The model under review builds one solid part; all positions refer to its coordinate system, in mm. A direction names the side the tool comes from. Coordinates: 2 decimals unless noted, no trailing zeros. Order: outer loops, then holes, each group sorted by start corner. A loop starts at its lowest first (then second) coordinate and runs counter-clockwise, first axis right, second up. Notation, with made-up numbers: (75.5, 33.5) -> (89.5, 33.5) arc R26 cw to (89.5, 59.5) -> close; hole circle Ø4 at (10.5, 60.25). An arc over 180 degrees is marked (long way). Use one line per item in the form item = value. Start each with the question number.
(1) Mouldability with a two-part tool opening along X and no side actions: class faces 1 (the flat face through (-8.72, -8.47, -1.57)), 2 (the flat face through (8.47, -8.72, -1.57)), 3 (the flat face through (-6.26, -1.95, -1.57)) as +X half, -X half, draft (parallel to the pull), parting line (faces both ways), or undercut.
(2) Insertion check: pin 1 Ø5 at (x, y) = (5, -14.5) entering from +Z; pin 2 Ø1.5 at (y, z) = (1.5, 22.5) entering from +X; pin 3 Ø4 at (y, z) = (-1, 6.5) entering from +X. Each pin has a flat end and moves straight along its axis. Give the tip position at first contact, or say it passes through.
(3) Take a section at A-A (y = -3). State the section outline as (x, z) points (3 decimals).
(4) Wall thickness on line 1 along Z through (x, y) = (-13, 2.5) (3 decimals); line 2 along X through (y, z) = (-0.5, 25.5); line 3 along Y through (x, z) = (9.5, 35): over which ranges is each line inside the solid? List them lowest first.
(5) Take a section at B-B (y = 2.5). State the section outline as (x, z) points (3 decimals), then the cut area to 3 significant figures.
(6) For faces 4 (the flat face through (6.44, -1.77, -1.57)), 5 (the flat face through (-14.91, 2.28, -1.57)), list the 3-axis set-ups (+Z, -Z, +X, -X, +Y, -Y) from which the entire face can be reached by the end or side of a thin tool; tool diameter is ignored.
(7) Take a section at C-C (x = 15). State the section outline as (y, z) points (3 decimals).
(8) Take a section at D-D (y = -15.25). State the section outline as (x, z) points (3 decimals).
```python
from build123d import *

# Parameters (mm, degrees)
F1_R     = 1.651
F4_DEPTH = 3.175


with BuildPart() as f2:
    # F2: sweep along a path in F0
    with BuildLine(Plane.XZ) as f2_path:
        Line((-12.7, 0), (-7.687481, 40.823691))
        ThreePointArc((-7.687481, 40.823691), (0, 47.625), (7.687481, 40.823691))
        Line((7.687481, 40.823691), (12.7, 0))
    # F1 (on Top) → F2 (sweep)
    with BuildSketch(Plane.XY):
        with Locations((-12.7, 0)):
            Circle(F1_R)
    sweep(path=f2_path.line)

    # F3 (on Top) → F4 (join)
    with BuildSketch(Plane.XY):
        Polygon((-17.190128, 0), (0, -17.190128), (0, -8.209872), (-12.7, 4.490128), align=None)
        Polygon((0, -8.209872), (0, -17.190128), (17.190128, 0), (12.7, 4.490128), align=None)
    extrude(amount=-F4_DEPTH)


solid = f2.part
```
Findings:
q1.face_1 = -X half
q1.face_2 = +X half
q1.face_3 = undercut
q2.pin_1 = 0
q2.pin_2 = 11.42
q2.pin_3 = 13.77
q3.outline = (-14.19, -3.175) -> (-5.21, -3.175) -> (-5.21, 0) -> (-14.19, 0) -> close; (5.21, -3.175) -> (14.19, -3.175) -> (14.19, 0) -> (5.21, 0) -> close
q4.line_1 = -3.175 to 0
q4.line_2 = -11.14 to -8, 8 to 11.14
q4.line_3 = -1.23 to 1.23
q5.outline = (-14.69, -3.175) -> (-10.71, -3.175) -> (-10.71, 0) -> (-14.69, 0) -> close; (10.71, -3.175) -> (14.69, -3.175) -> (14.69, 0) -> (10.71, 0) -> close
q5.area = 25.3 mm²
q6.face_4 = -Z, +Y
q6.face_5 = +Z, -Z, -X, +Y
q7.outline = (-2.19, -3.175) -> (2.19, -3.175) -> (2.19, 0) -> (-2.19, 0) -> close
q8.outline = (-1.94, -3.175) -> (1.94, -3.175) -> (1.94, 0) -> (-1.94, 0) -> close
